from build123d import *

# Parameters (mm, degrees)
SKETCH_1_R          = 18.3
EXTRUDE_1_DEPTH     = 21.5
SKETCH_2_R          = 1.5
CUT_EXTRUDE_1_DEPTH = 5
SKETCH_3_R          = 6
EXTRUDE_2_DEPTH     = 6
SKETCH_4_R          = 3
EXTRUDE_3_DEPTH     = 13.8
CUT_EXTRUDE_START   = -11.5
CUT_EXTRUDE_2_DEPTH = 11.5
SKETCH_6_R          = 16.4
EXTRUDE_4_DEPTH     = 23
SKETCH_7_R          = 15
EXTRUDE_5_DEPTH     = 1
SKETCH_8_R          = 3
EXTRUDE_6_DEPTH     = 4
SKETCH_9_W          = 12.161670498
SKETCH_9_H          = 4.500444444
EXTRUDE_7_DEPTH     = 7.9
SKETCH_10_W         = 1.2
SKETCH_10_H         = 2.711111112
EXTRUDE_8_DEPTH     = 4
SKETCH_11_W         = 10.179858782
SKETCH_11_H         = 6.369590588
CUT_EXTRUDE_3_DEPTH = 6


with BuildPart() as part:
    # 草图1 → 凸台-拉伸1 (new body)
    with BuildSketch(Plane.XY):
        Circle(SKETCH_1_R)
    extrude(amount=EXTRUDE_1_DEPTH)

    # 草图2 → 切除-拉伸1 (cut)
    with BuildSketch(Plane.XY.offset(21.5)):
        with Locations((0, 15.5)):
            Circle(SKETCH_2_R)
        with Locations((13.423393759, 7.75)):
            Circle(SKETCH_2_R)
        with Locations((13.423393759, -7.75)):
            Circle(SKETCH_2_R)
        with Locations((0, -15.5)):
            Circle(SKETCH_2_R)
        with Locations((-13.423393759, -7.75)):
            Circle(SKETCH_2_R)
        with Locations((-13.423393759, 7.75)):
            Circle(SKETCH_2_R)
    extrude(amount=-CUT_EXTRUDE_1_DEPTH, mode=Mode.SUBTRACT)

    # 草图3 → 凸台-拉伸2 (add)
    with BuildSketch(Plane.XY.offset(21.5)):
        with Locations((7.3, 0)):
            Circle(SKETCH_3_R)
    extrude(amount=EXTRUDE_2_DEPTH)

    # 草图4 → 凸台-拉伸3 (add)
    with BuildSketch(Plane.XY.offset(27.5)):
        with Locations(Location((7.3, 0, 0), (0, 0, 180))):
            Circle(SKETCH_4_R)
    extrude(amount=EXTRUDE_3_DEPTH)

    # 草图5 → 切除-拉伸2 (cut)
    with BuildSketch(Plane.XY.offset(41.3).offset(CUT_EXTRUDE_START)):
        with BuildLine():
            Line((5.641687605, 2.5), (8.958312395, 2.5))
            ThreePointArc((8.958312395, 2.5), (7.3, 3), (5.641687605, 2.5))
        make_face()
    extrude(amount=CUT_EXTRUDE_2_DEPTH, mode=Mode.SUBTRACT)

    # 草图6 → 凸台-拉伸4 (add)
    with BuildSketch(Plane(origin=(0, 0, 0), x_dir=(-1, 0, 0), z_dir=(0, 0, -1))):
        Circle(SKETCH_6_R)
    extrude(amount=EXTRUDE_4_DEPTH)

    # 草图7 → 凸台-拉伸5 (add)
    with BuildSketch(Plane(origin=(0, 0, -23), x_dir=(-1, 0, 0), z_dir=(0, 0, -1))):
        Circle(SKETCH_7_R)
    extrude(amount=EXTRUDE_5_DEPTH)

    # 草图8 → 凸台-拉伸6 (add)
    with BuildSketch(Plane(origin=(0, 0, -24), x_dir=(-1, 0, 0), z_dir=(0, 0, -1))):
        Circle(SKETCH_8_R)
    extrude(amount=EXTRUDE_6_DEPTH)

    # 草图9 → 凸台-拉伸7 (add)
    with BuildSketch(Plane(origin=(0, 0, -24), x_dir=(-1, 0, 0), z_dir=(0, 0, -1))):
        with Locations((0, -11.791042912)):
            Rectangle(SKETCH_9_W, SKETCH_9_H)
    extrude(amount=EXTRUDE_7_DEPTH)

    # 草图10 → 凸台-拉伸8 (add)
    with BuildSketch(Plane(origin=(0, 0, -24), x_dir=(-1, 0, 0), z_dir=(0, 0, -1))):
        with Locations((-5.289655172, 0)):
            Rectangle(SKETCH_10_W, SKETCH_10_H)
        with Locations((5.835249042, 0)):
            Rectangle(SKETCH_10_W, SKETCH_10_H)
    extrude(amount=EXTRUDE_8_DEPTH)

    # 草图11 → 切除-拉伸3 (cut)
    with BuildSketch(Plane(origin=(0, 0, -31.9), x_dir=(-1, 0, 0), z_dir=(0, 0, -1))):
        with Locations((0, -14.041265134)):
            Rectangle(SKETCH_11_W, SKETCH_11_H)
    extrude(amount=-CUT_EXTRUDE_3_DEPTH, mode=Mode.SUBTRACT)


solid = part.part
Input: part model. Units: mm. Frame: model coordinates. A direction names the side the tool comes from. Coordinates: 2 decimals unless noted, no trailing zeros. Write each loop counter-clockwise with the first axis right and the second up, starting at its lowest first coordinate (ties: lowest second). Pieces come first, ordered by that corner, then holes. Notation, with made-up numbers: M 87,21 L 136,21 A30 cw 136,44 Z; hole C 56,-19.5 d1. An arc over 180 degrees is marked long. Answer as a JSON object with one key per item and string values. Group by question number.
(1) Section B-B on y = 7.75. Output: boundary loops of the cut face in (x, z).
(2) Section A-A on z = 19. Output: boundary loops of the cut face in (x, y), plus the area to 3 significant figures.
(3) Ray query, line 1 along Y through (x, z) = (0, 18.4); line 2 along Z through (x, y) = (2.5, 1.5); line 3 along Z through (x, y) = (1, -11.5). Return the intervals inside material, ascending. Write a range as [from, to].
(4) Section C-C on x = 7.3. Output: boundary loops of the cut face in (y, z), plus the area to 3 significant figures.
(5) Mould query, pull axis X, two halves, no side actions, for faces 1 (the face through (13, -8, 16.5)), 2 (the face through (-6.081, -12, -28)), 3 (the face through (7, 0, 41.3)). Classes: pulls with the +X half, pulls with the -X half, needs draft (parallel to the pull), parting line crosses it, or undercut.
(6) Set-up query: faces 4 (the face through (3, 0, -26)), 5 (the face through (4.69, 0, -26)), 6 (the face through (6.081, -12, -28)), 7 (the face through (0, -14.041, -25)), 8 (the face through (13.023, 1.802, 24.458)). Return all of +Z, -Z, +X, -X, +Y, -Y with unobstructed straight access to the full face (end or side cutting, diameter ignored); none if empty.
(7) Contact query for flat-ended pins moving along their axis: P1, Ø2, axis at y = 7.5, z = 16.5, coming from the +X side; P2, Ø0.9, axis at x = 0.5, y = 16, coming from the +Z side; P3, Ø8.5, axis at x = -6.5, y = 2, coming from the -Z side; P4, Ø2, axis at y = 4, z = 33, coming from the -X side. Output: stop coordinate, or through.
(8) Section D-D on z = 6. Output: boundary loops of the cut face in (x, y).
Result set:
{
 "1": {"outline": "M -16.58,0 L -14.45,0 L -14.45,-23 L -12.84,-23 L -12.84,-24 L 12.84,-24 L 12.84,-23 L 14.45,-23 L 14.45,0 L 16.58,0 L 16.58,21.5 L 14.92,21.5 L 14.92,16.5 L 11.92,16.5 L 11.92,21.5 L -11.92,21.5 L -11.92,16.5 L -14.92,16.5 L -14.92,21.5 L -16.58,21.5 Z"},
 "2": {"outline": "C 0,0 d36.6; hole C -13.42,-7.75 d3; hole C -13.42,7.75 d3; hole C 0,-15.5 d3; hole C 0,15.5 d3; hole C 13.42,-7.75 d3; hole C 13.42,7.75 d3", "area": "1,010 mm2"},
 "3": {"line 1": "y = [-18.3, -17], [-14, 14], [17, 18.3]", "line 2": "z = [-28, 27.5]", "line 3": "z = [-25.9, 21.5]"},
 "4": {"outline": "M -16.78,0 L -14.69,0 L -14.69,-23 L -13.1,-23 L -13.1,-24 L 13.1,-24 L 13.1,-23 L 14.69,-23 L 14.69,0 L 16.78,0 L 16.78,21.5 L 6,21.5 L 6,27.5 L 3,27.5 L 3,29.8 L 2.5,29.8 L 2.5,41.3 L -3,41.3 L -3,27.5 L -6,27.5 L -6,21.5 L -16.78,21.5 Z", "area": "1,570 mm2"},
 "5": {"face 1": "undercut", "face 2": "pulls with the -X half", "face 3": "needs draft"},
 "6": {"face 4": "-Z", "face 5": "-Z, +Y", "face 6": "-Z, +X, +Y, -Y", "face 7": "-Z, +X, -X, -Y", "face 8": "+Z"},
 "7": {"P1": "stops at x = 17.11", "P2": "stops at z = 16.5", "P3": "stops at z = -28", "P4": "passes through"},
 "8": {"outline": "C 0,0 d36.6"}
}
